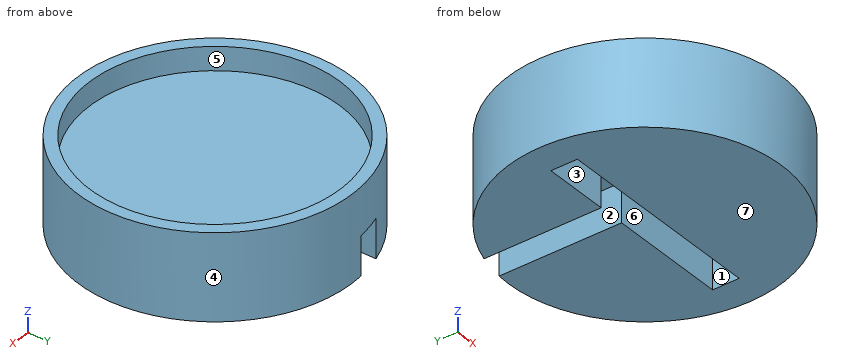
```python
from build123d import *

# Parameters (mm, degrees)
F0_R     = 17.5
F1_DEPTH = 11
F2_R     = 16
F3_DEPTH = 3
F4_W     = 13.5
F4_H     = 1.7
F5_DEPTH = 5


with BuildPart() as f1:
    # F0 (on Top) → F1 (new body)
    with BuildSketch(Plane.XY):
        Circle(F0_R)
    extrude(amount=F1_DEPTH)

    # F2 (on face) → F3 (cut)
    with BuildSketch(Plane.XY.offset(11)):
        Circle(F2_R)
    extrude(amount=-F3_DEPTH, mode=Mode.SUBTRACT)

    # F4 (on face) → F5 (cut)
    with BuildSketch(Plane(origin=(0, 0, 0), x_dir=(1, 0, 0), z_dir=(0, 0, -1))):
        with BuildLine():
            Line((-1.7, -17.4172328457), (-1.7, -1.7))
            Line((-1.7, -1.7), (-5.1, -1.7))
            Line((-5.1, -1.7), (-5.1, -16.7403703663))
            ThreePointArc((-5.1, -16.7403703663), (-3.4168019703, -17.1632008756), (-1.7, -17.4172328457))
        make_face()
        Polygon((0, -1.7), (0, 0), (-13.5, 0), (-13.5, -1.7), (-5.1, -1.7), (-1.7, -1.7), align=None)
        Polygon((13.5, 0), (0, 0), (0, -1.7), (1.7, -1.7), (13.5, -1.7), align=None)
        with Locations((6.75, 0.85)):
            Rectangle(F4_W, F4_H)
        with Locations((-6.75, 0.85)):
            Rectangle(F4_W, F4_H)
    extrude(amount=-F5_DEPTH, mode=Mode.SUBTRACT)


solid = f1.part
```
Model file for the job. Use its own axes, mm. Face numbers are marked on the shaded views. A direction names the side the tool comes from. Coordinates: 2 decimals unless noted, no trailing zeros. Order: outer loops, then holes, each group sorted by start corner. A loop starts at its lowest first (then second) coordinate and runs counter-clockwise, first axis right, second up. Notation, with made-up numbers: M -32.75,-11 L 5.25,-11 A17 ccw 5.25,8 Z; hole C 66.25,34.5 d2. An arc over 180 degrees is marked long. Answer as CSV lines item,"result".
(1) Band-saw the part on D-D, the plane z = 8.5. List the corners of the cut face in (x, y).
Geometry says:
outline,"C 0,0 d35; hole C 0,0 d32"
(2) Wall check: line 1 along Y through (x, z) = (0, 10.1); line 2 along Z through (x, y) = (-10, -1); line 3 along X through (y, z) = (12, 9.25). Give the ranges that are in metal, low to high.
Geometry says:
line 1,"y = -17.5 to -16, 16 to 17.5"
line 2,"z = 5 to 8"
line 3,"x = -12.74 to -10.58, 10.58 to 12.74"
(3) Band-saw the part on A-A, the plane x = 0. List the corners of the cut face in (y, z), then the cut area to 3 significant figures.
Geometry says:
outline,"M -17.5,0 L -1.7,0 L -1.7,5 L 1.7,5 L 1.7,0 L 17.5,0 L 17.5,11 L 16,11 L 16,8 L -16,8 L -16,11 L -17.5,11 Z"
area,"272 mm2"
(4) Band-saw the part on B-B, the plane z = 2.5. List the corners of the cut face in (x, y), then the cut area to 3 significant figures.
Geometry says:
outline,"M -13.5,-1.7 L -13.5,1.7 L -5.1,1.7 L -5.1,16.74 A17.5 ccw long -1.7,17.42 L -1.7,1.7 L 13.5,1.7 L 13.5,-1.7 Z"
area,"818 mm2"
(5) 3-axis set-ups, long thin cutter, end or side, ignore diameter. For the marked faces 5, 6 and 7: which of +Z, -Z, +X, -X, +Y, -Y reach the whole face in a straight line?
Geometry says:
face 5,"+Z"
face 6,"-Z"
face 7,"-Z, +X, -X, +Y, -Y"
(6) Pull direction Y, two halves, no side cores. Call the marked faces 1, 2, 3 and 4: +Y half, -Y half, draft (parallel to the pull), parting line (faces both ways), or undercut.
Geometry says:
face 1,"undercut"
face 2,"draft"
face 3,"undercut"
face 4,"parting line"
(7) Flat gauge pins, fed straight in: pin 1 (2.5 mm diameter, centred on y = 10.5, z = 3.5, fed in from -X); pin 2 (5.5 mm diameter, centred on x = -10.5, z = 2.5, fed in from -Y); pin 3 (2.5 mm diameter, centred on x = 2.5, z = 3, fed in from +Y). Where does each tip first touch, or does it go through?
Geometry says:
pin 1,"stops at x = -14.86"
pin 2,"stops at y = -15.69"
pin 3,"stops at y = 17.46"
(8) Band-saw the part on C-C, the plane y = 0. List the corners of the cut face in (x, z).
Geometry says:
outline,"M -17.5,0 L -13.5,0 L -13.5,5 L 13.5,5 L 13.5,0 L 17.5,0 L 17.5,11 L 16,11 L 16,8 L -16,8 L -16,11 L -17.5,11 Z"
